CAD build for the part. Positions are in the model's coordinates, mm. Face numbers are marked on the shaded views. Round coordinates to 2 decimals unless told otherwise and drop trailing zeros. Loops run counter-clockwise (first coordinate to the right, second up) from the corner with the lowest first, then second, coordinate; pieces in that order, holes last.
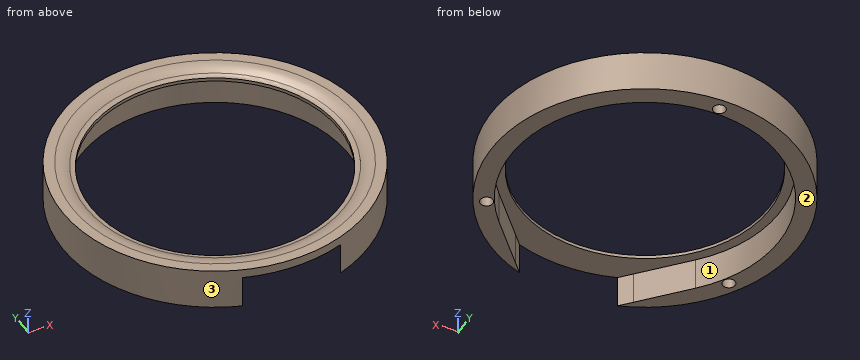
from build123d import *

# Parameters (mm, degrees)
CUT_EXTRUDE_2_DEPTH      = 1
CUT_EXTRUDE_2_DEPTH_BACK = 32.472368834
SKETCH_3_R               = 0.9
CUT_EXTRUDE_3_DEPTH      = 4
PATTERN_CIRCULAR_1_COUNT = 3


with BuildPart() as part:
    # ｽｹｯﾁ1 → 回転1 (revolve)
    with BuildSketch(Plane(origin=(0, 0, 0), x_dir=(1, 0, 0), z_dir=(0, 1, 0)), mode=Mode.PRIVATE) as revolve_1_sk:
        with BuildLine():
            Line((17.95, -1.5), (17.95, 3.7))
            Line((17.95, 3.7), (22.1, 3.7))
            Line((22.1, 3.7), (22.1, -2.3))
            Line((22.1, -2.3), (20.6, -2.3))
            ThreePointArc((20.6, -2.3), (19.598521282, -2.152129029), (18.682513342, -1.721136103))
            ThreePointArc((18.682513342, -1.721136103), (18.332582335, -1.556489289), (17.95, -1.5))
        make_face()
    revolve(revolve_1_sk.sketch.rotate(Axis((0, 0, -23.242467286), (0, 0, 1)), 180), axis=Axis((0, 0, -23.242467286), (0, 0, 1)))

    # ｽｹｯﾁ2 → ｶｯﾄ - 押し出し2 (cut, two sides: drawn at the far end of the back side and taken through both)
    with BuildSketch(Plane.XY.offset(-CUT_EXTRUDE_2_DEPTH_BACK)):
        with BuildLine():
            Line((-14.300155258, -13.03564573), (-8.573902611, -19.317367678))
            Line((-8.573902611, -19.317367678), (-4.755467222, -23.5062065))
            Line((-4.755467222, -23.5062065), (4.755467222, -23.5062065))
            Line((4.755467222, -23.5062065), (8.573902611, -19.317367678))
            Line((8.573902611, -19.317367678), (14.300155258, -13.03564573))
            ThreePointArc((14.300155258, -13.03564573), (0, 19.35), (-14.300155258, -13.03564573))
        make_face()
    extrude(amount=CUT_EXTRUDE_2_DEPTH + CUT_EXTRUDE_2_DEPTH_BACK, mode=Mode.SUBTRACT)

    # ｽｹｯﾁ3 → ｶｯﾄ - 押し出し3 (cut)
    with BuildSketch(Plane(origin=(0, 0, -3.7), x_dir=(-1, 0, 0), z_dir=(0, 0, -1))):
        with Locations((0, 20.35)):
            Circle(SKETCH_3_R)
    cut_extrude_3 = extrude(amount=-CUT_EXTRUDE_3_DEPTH, mode=Mode.SUBTRACT)

    # 円形ﾊﾟﾀｰﾝ1: ｶｯﾄ - 押し出し3 ×3 about axis
    pattern_circular_1_axis = Axis((0, 0, 0), (0, 0, 1))
    for i in range(1, PATTERN_CIRCULAR_1_COUNT):
        add(cut_extrude_3.rotate(pattern_circular_1_axis, i * 360 / PATTERN_CIRCULAR_1_COUNT), mode=Mode.SUBTRACT)


solid = part.part
Item 1: Cut at C-C (z = -1.25). List the corners of the cut face in (x, y) (3 decimals).
Verdict:
outline: (-14.3, -13.036) arc R19.35 cw (long way) to (14.3, -13.036) - (7.108, -20.926) arc R22.1 ccw (long way) to (-7.108, -20.926) - close; hole circle Ø1.8 at (-17.624, -10.175); hole circle Ø1.8 at (0, 20.35); hole circle Ø1.8 at (17.624, -10.175)
Item 2: Mould opens along Y. For the marked faces 1, 2 and 3 say: released by +Y, released by -Y, zero draft, split by the parting line, or undercut.
Verdict:
face 1: undercut
face 2: zero draft
face 3: split by the parting line
Item 3: Cut at B-B (x = 0). List the corners of the cut face in (y, z), plus the area to 3 significant figures.
Verdict:
outline: (-22.1, 1) - (-17.95, 1) - (-17.95, 1.5) arc R1.32 cw to (-18.68, 1.72) arc R3.47 ccw to (-20.6, 2.3) - (-22.1, 2.3) - close; (17.95, 1) - (19.35, 1) - (19.35, -3.7) - (19.45, -3.7) - (19.45, 0.3) - (21.25, 0.3) - (21.25, -3.7) - (22.1, -3.7) - (22.1, 2.3) - (20.6, 2.3) arc R3.47 ccw to (18.68, 1.72) arc R1.32 cw to (17.95, 1.5) - close
area: 14.7 mm2
Item 4: Cut at A-A (y = 0). List the corners of the cut face in (x, z), plus the area to 3 significant figures.
Verdict:
outline: (-22.1, -3.7) - (-19.35, -3.7) - (-19.35, 1) - (-17.95, 1) - (-17.95, 1.5) arc R1.32 cw to (-18.68, 1.72) arc R3.47 ccw to (-20.6, 2.3) - (-22.1, 2.3) - close; (17.95, 1) - (19.35, 1) - (19.35, -3.7) - (22.1, -3.7) - (22.1, 2.3) - (20.6, 2.3) arc R3.47 ccw to (18.68, 1.72) arc R1.32 cw to (17.95, 1.5) - close
area: 34.9 mm2
Item 5: Flat gauge pins, fed straight in: P1, Ø1.4, axis at x = 0, y = 20.35, coming from the -Z side; P2, Ø3, axis at x = -6, z = -1.5, coming from the +Y side; P3, Ø1, axis at x = -0.5, z = -3, coming from the -Y side. Where does each tip first touch, or does it go through?
Verdict:
P1: stops at z = 0.3
P2: stops at y = 21.64
P3: stops at y = 19.32
Item 6: Wall check: L1, parallel to X at y = -10, z = -1.75; L2, parallel to Y at x = -17.5, z = -3.5; L3, parallel to Z at x = -18, y = 9.5. Give the ranges that are in metal, low to high.
Verdict:
L1: x = -19.71 to -18.51, -16.74 to -16.57, 16.57 to 16.74, 18.51 to 19.71
L2: y = -13.5 to -11.07, -9.28 to -8.26, 8.26 to 13.5
L3: z = -3.7 to 2.29
